Check sheet for the drawn part. Datum: minimum x, y, z corner. Units: mm. A direction names the side the tool comes from. Give positions to 0.01 mm unless a question says otherwise; leave off trailing zeros. Write each loop counter-clockwise with the first axis right and the second up, starting at its lowest first coordinate (ties: lowest second). Pieces come first, ordered by that corner, then holes. Notation, with made-up numbers: M -17,58.5 L 41,58.5 A25 ccw 41,92.5 Z; hole C -23.75,0.25 d4. An arc over 180 degrees is marked long. Write item = value, one per line.
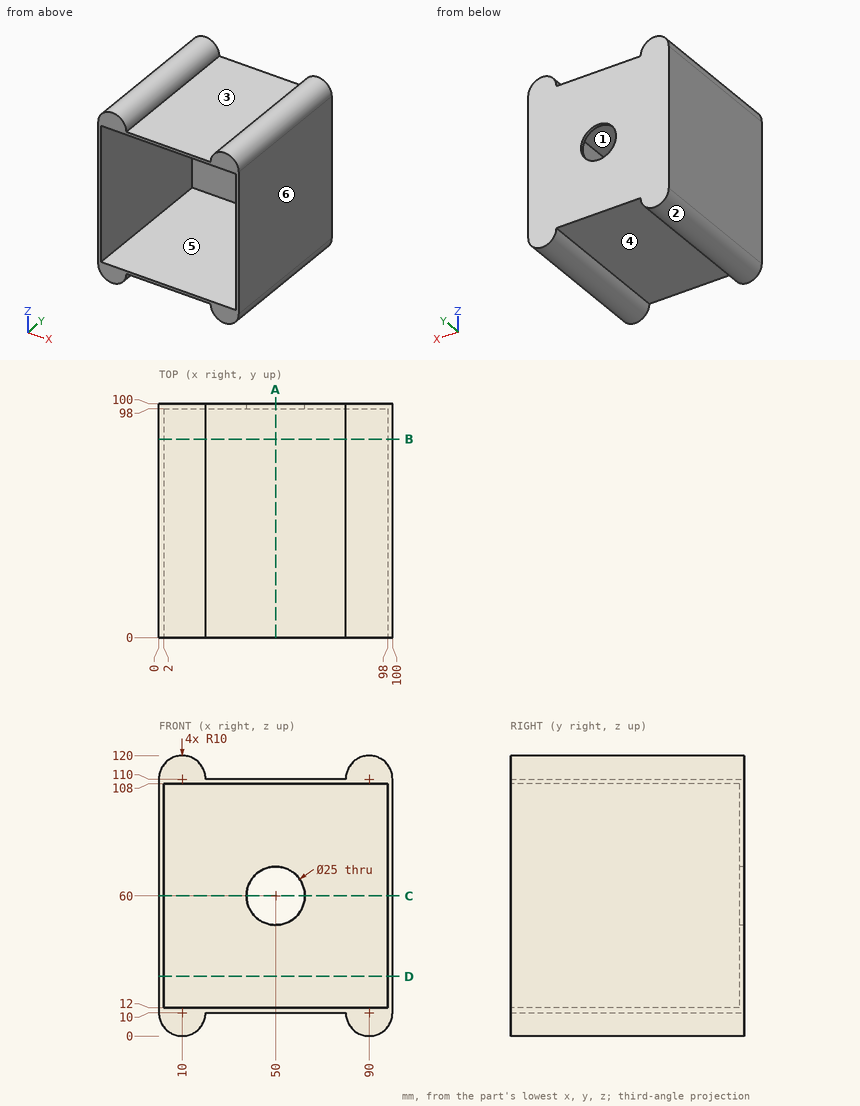
1) Depth check by flat-ended pin: P1, Ø10, axis at x = 55.5, y = 11.5, coming from the -Z side; P2, Ø18, axis at x = 41.5, y = 51.5, coming from the +Z side; P3, Ø10, axis at x = 23, z = 31, coming from the -Y side; P4, Ø15, axis at x = 50, z = 60, coming from the -Y side. Enter the tip coordinate at first touch or a pass-through.
From the geometry:
P1 = 10
P2 = 110
P3 = 98
P4 = through
2) Tool access check on the marked faces 4, 5 and 6. Record the directions out of +Z, -Z, +X, -X, +Y, -Y that give a thin tool (end or side, any length) a straight path to the whole face; none if there is none.
From the geometry:
face_4 = -Z, +Y, -Y
face_5 = -Y
face_6 = +Z, -Z, +X, +Y, -Y
3) Material ranges on probe 1 along X at (y, z) = (59, 12.5); probe 2 along Z at (x, y) = (69, 67); probe 3 along Z at (x, y) = (50, 99.3), recorded low to high. Write a range as from..to.
From the geometry:
probe_1 = 0..2, 98..100
probe_2 = 10..12, 108..110
probe_3 = 10..47.5, 72.5..110
4) Cross-section at B-B on y = 85. Record the boundary of the cut face in (x, z).
From the geometry:
outline = M 0,10 A10 ccw 20,10 L 80,10 A10 ccw 100,10 L 100,110 A10 ccw 80,110 L 20,110 A10 ccw 0,110 Z; hole M 2,12 L 98,12 L 98,108 L 2,108 Z
5) Cross-section at D-D on z = 25.5. Record the boundary of the cut face in (x, y), plus the area to 3 significant figures.
From the geometry:
outline = M 0,0 L 2,0 L 2,98 L 98,98 L 98,0 L 100,0 L 100,100 L 0,100 Z
area = 592 mm^2
6) Draft check along Z on the marked faces 1, 2 and 3. Enter one of: +Z half, -Z half, draft (parallel to the pull), parting line (faces both ways), or undercut.
From the geometry:
face_1 = undercut
face_2 = -Z half
face_3 = +Z half
7) Cross-section at A-A on x = 50. Record the boundary of the cut face in (y, z).
From the geometry:
outline = M 0,10 L 100,10 L 100,47.5 L 98,47.5 L 98,12 L 0,12 Z; M 0,108 L 98,108 L 98,72.5 L 100,72.5 L 100,110 L 0,110 Z
8) Cross-section at C-C on z = 60. Record the boundary of the cut face in (x, y).
From the geometry:
outline = M 0,0 L 2,0 L 2,98 L 37.5,98 L 37.5,100 L 0,100 Z; M 62.5,98 L 98,98 L 98,0 L 100,0 L 100,100 L 62.5,100 Z
